Build history of the part. All positions in model axes, mm. Give positions to 0.01 mm unless a question says otherwise; leave off trailing zeros. Order: outer loops, then holes, each group sorted by start corner. A loop starts at its lowest first (then second) coordinate and runs counter-clockwise, first axis right, second up. Notation, with made-up numbers: (62.25, -6) - (70.25, -6) arc R27 ccw to (70.25, 23) - close; hole circle Ø6 at (19.25, 72.5). An arc over 180 degrees is marked (long way). One line per item, written item: value.
```python
from build123d import *

# Parameters (mm, degrees)
SKETCH1_R           = 63.5
SKETCH1_R_2         = 38.1
BOSS_EXTRUDE1_DEPTH = 2.750000088
SKETCH2_W           = 9.380000036
SKETCH2_H           = 2.605000124
SKETCH2_W_2         = 2.605000124
SKETCH2_H_2         = 9.380000036
CUT_EXTRUDE1_DEPTH  = 90.844657607


with BuildPart() as part:
    # Sketch1 → Boss-Extrude1 (new body)
    with BuildSketch(Plane(origin=(0, 0, 0), x_dir=(0, 1, 0), z_dir=(0, 0, 1))):
        with Locations(Location((0, 0, 0), (0, 0, 270))):
            Circle(SKETCH1_R)
        with Locations(Location((0, 0, 0), (0, 0, 270))):
            Circle(SKETCH1_R_2, mode=Mode.SUBTRACT)
    extrude(amount=BOSS_EXTRUDE1_DEPTH)

    # Sketch2 → Cut-Extrude1 (cut, through all)
    with BuildSketch(Plane.XY.offset(2.750000088)):
        with Locations((49.055203892, 0)):
            Rectangle(SKETCH2_W, SKETCH2_H)
        with Locations((0, 49.055203892)):
            Rectangle(SKETCH2_W_2, SKETCH2_H_2)
        with Locations((0, -49.055203892)):
            Rectangle(SKETCH2_W_2, SKETCH2_H_2)
        with Locations((-49.055203892, 0)):
            Rectangle(SKETCH2_W, SKETCH2_H)
    extrude(amount=-CUT_EXTRUDE1_DEPTH, mode=Mode.SUBTRACT)


solid = part.part
```
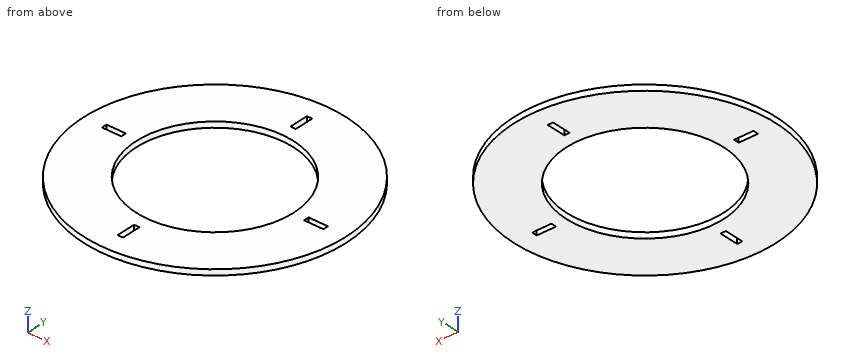
(1) Pin check, flat tips, straight feed: P1, Ø0.8, axis at x = 0.5, z = 1, coming from the +Y side; P2, Ø1.4, axis at x = -51, z = 2, coming from the -Y side; P3, Ø1.4, axis at y = 47.5, z = 1, coming from the -X side. Stop position of each tip, or through.
Completed:
P1: y = 63.5
P2: y = -38.76
P3: x = -42.92
(2) Slice it at A-A, the plane z = 1.95. Give the cut face in (x, y).
Completed:
outline: circle Ø127 at (0, 0); hole (-53.75, -1.3) - (-44.37, -1.3) - (-44.37, 1.3) - (-53.75, 1.3) - close; hole circle Ø76.2 at (0, 0); hole (-1.3, -53.75) - (1.3, -53.75) - (1.3, -44.37) - (-1.3, -44.37) - close; hole (-1.3, 44.37) - (1.3, 44.37) - (1.3, 53.75) - (-1.3, 53.75) - close; hole (44.37, -1.3) - (53.75, -1.3) - (53.75, 1.3) - (44.37, 1.3) - close
(3) Slice it at B-B, the plane y = -5.5. Give the cut face in (x, z).
Completed:
outline: (-63.26, 0) - (-37.7, 0) - (-37.7, 2.75) - (-63.26, 2.75) - close; (37.7, 0) - (63.26, 0) - (63.26, 2.75) - (37.7, 2.75) - close
(4) Drill centre lines: line 1 (Y direction, x = 0, z = 0.6); line 2 (X direction, y = -5.5, z = 2.35); line 3 (X direction, y = 4, z = 1.9). Where is each one in solid material? Low to high.
Completed:
line 1: -63.5 to -53.75, -44.37 to -38.1, 38.1 to 44.37, 53.75 to 63.5
line 2: -63.26 to -37.7, 37.7 to 63.26
line 3: -63.37 to -37.89, 37.89 to 63.37
(5) Slice it at C-C, the plane x = 7. Give the cut face in (y, z), and give its area (3 significant figures).
Completed:
outline: (-63.11, 0) - (-37.45, 0) - (-37.45, 2.75) - (-63.11, 2.75) - close; (37.45, 0) - (63.11, 0) - (63.11, 2.75) - (37.45, 2.75) - close
area: 141 mm²
